```python
from build123d import *

# Parameters (mm, degrees)
BOSS_EXTRUDE1_DEPTH = 1.6


with BuildPart() as part:
    # Sketch2 → Boss-Extrude1 (new body)
    with BuildSketch(Plane.XY):
        with BuildLine():
            Line((-47.121320344, 0.878679656), (-45.878679656, 2.121320344))
            ThreePointArc((-45.878679656, 2.121320344), (-44.90540961, 2.771638598), (-43.757359313, 3))
            Line((-43.757359313, 3), (43.757359313, 3))
            ThreePointArc((43.757359313, 3), (44.90540961, 2.771638598), (45.878679656, 2.121320344))
            Line((45.878679656, 2.121320344), (47.121320344, 0.878679656))
            ThreePointArc((47.121320344, 0.878679656), (48.09459039, 0.228361402), (49.242640687, 0))
            Line((49.242640687, 0), (52, 0))
            ThreePointArc((52, 0), (54.121320344, 0.878679656), (55, 3))
            Line((55, 3), (55, 55))
            ThreePointArc((55, 55), (54.121320344, 57.121320344), (52, 58))
            Line((52, 58), (49.367496998, 58))
            ThreePointArc((49.367496998, 58), (48.717977945, 57.852081728), (48.196559873, 57.4375))
            ThreePointArc((48.196559873, 57.4375), (40, 53.5), (31.803440127, 57.4375))
            ThreePointArc((31.803440127, 57.4375), (31.282022055, 57.852081728), (30.632503002, 58))
            Line((30.632503002, 58), (29.367496998, 58))
            ThreePointArc((29.367496998, 58), (28.717977945, 57.852081728), (28.196559873, 57.4375))
            ThreePointArc((28.196559873, 57.4375), (20, 53.5), (11.803440127, 57.4375))
            ThreePointArc((11.803440127, 57.4375), (11.282022055, 57.852081728), (10.632503002, 58))
            Line((10.632503002, 58), (9.367496998, 58))
            ThreePointArc((9.367496998, 58), (8.717977945, 57.852081728), (8.196559873, 57.4375))
            ThreePointArc((8.196559873, 57.4375), (0, 53.5), (-8.196559873, 57.4375))
            ThreePointArc((-8.196559873, 57.4375), (-8.717977945, 57.852081728), (-9.367496998, 58))
            Line((-9.367496998, 58), (-10.632503002, 58))
            ThreePointArc((-10.632503002, 58), (-11.282022055, 57.852081728), (-11.803440127, 57.4375))
            ThreePointArc((-11.803440127, 57.4375), (-20, 53.5), (-28.196559873, 57.4375))
            ThreePointArc((-28.196559873, 57.4375), (-28.717977945, 57.852081728), (-29.367496998, 58))
            Line((-29.367496998, 58), (-30.632503002, 58))
            ThreePointArc((-30.632503002, 58), (-31.282022055, 57.852081728), (-31.803440127, 57.4375))
            ThreePointArc((-31.803440127, 57.4375), (-40, 53.5), (-48.196559873, 57.4375))
            ThreePointArc((-48.196559873, 57.4375), (-48.717977945, 57.852081728), (-49.367496998, 58))
            Line((-49.367496998, 58), (-52, 58))
            ThreePointArc((-52, 58), (-54.121320344, 57.121320344), (-55, 55))
            Line((-55, 55), (-55, 3))
            ThreePointArc((-55, 3), (-54.121320344, 0.878679656), (-52, 0))
            Line((-52, 0), (-49.242640687, 0))
            ThreePointArc((-49.242640687, 0), (-48.09459039, 0.228361402), (-47.121320344, 0.878679656))
        make_face()
    extrude(amount=BOSS_EXTRUDE1_DEPTH)


solid = part.part
```
CAD build for the part. Positions are in the model's coordinates, mm. Round coordinates to 2 decimals unless told otherwise and drop trailing zeros. Order: outer loops, then holes, each group sorted by start corner. A loop starts at its lowest first (then second) coordinate and runs counter-clockwise, first axis right, second up. Notation, with made-up numbers: (-39.5, 56.25) -> (-12.5, 56.25) arc R12 cw to (-12.5, 71.25) -> close; hole circle Ø6 at (28, 66). An arc over 180 degrees is marked (long way). Write item = value, one per line.
(1) Cut at A-A (x = -33). Write the cut outline in (y, z), plus the area to 3 significant figures.
Answers follow:
outline = (3, 0) -> (56.17, 0) -> (56.17, 1.6) -> (3, 1.6) -> close
area = 85.1 mm²
(2) Cut at B-B (x = 15.5). Write the cut outline in (y, z).
Answers follow:
outline = (3, 0) -> (54.51, 0) -> (54.51, 1.6) -> (3, 1.6) -> close
(3) Drill centre lines: L1, parallel to Y at x = -30.5, z = 1.5; L2, parallel to Y at x = 14, z = 0.95. Where is each one in solid material? Low to high.
Answers follow:
L1 = 3 to 58
L2 = 3 to 55.38
(4) Pull direction X, two halves, no side cores. Call faces 1 (the cylindrical face through (40.1, 53.5, 0.8)), 2 (the cylindrical face through (54.1, 0.86, 0.79)), 3 (the cylindrical face through (-54.14, 0.9, 0.79)): +X half, -X half, draft (parallel to the pull), parting line (faces both ways), or undercut.
Answers follow:
face_1 = undercut
face_2 = +X half
face_3 = -X half
